Check sheet for the modelled part. Datum: model origin and axes. Units: mm. Round coordinates to 2 decimals unless told otherwise and drop trailing zeros. Order: outer loops, then holes, each group sorted by start corner. A loop starts at its lowest first (then second) coordinate and runs counter-clockwise, first axis right, second up. Notation, with made-up numbers: (-6, 22.5) -> (9, 22.5) arc R24 cw to (9, 32.5) -> close; hole circle Ø11 at (84, 21). An arc over 180 degrees is marked (long way). Answer in a Markdown table with one row per item. Add a question column.
1. Material ranges on L1, parallel to Y at x = -39.15, z = 0; L2, parallel to Z at x = -40.1, y = 9.75; L3, parallel to Y at x = -39.35, z = -31.5, recorded low to high. Write a range as from..to.
2. Sectioned sample at C-C, the plane z = 34. Count the separate pieces of the cut face and the enclosed holes in it, then the cut area to 3 significant figures.
3. Sectioned sample at A-A, the plane y = 9.75. Record the boundary of the cut face in (x, z), then the cut area to 3 significant figures.
4. Draft check along Y on faces 1 (the cylindrical face through (-39.532, 40.124, -47.641)), 2 (the cylindrical face through (-39.53, 4.97, 8.1)), 3 (the flat face through (-38.053, -2, -1)). Enter one of: +Y half, -Y half, draft (parallel to the pull), parting line (faces both ways), or undercut.
5. Depth check by flat-ended pin: P1, Ø4, axis at y = 3.39, z = -6.36, coming from the -X side; P2, Ø1.5, axis at x = -38.5, y = 29, coming from the -Z side; P3, Ø1.5, axis at x = -40.5, z = 26, coming from the +Y side. Enter the tip coordinate at first touch or a pass-through.
6. Sectioned sample at B-B, the plane z = 0. Record the boundary of the cut face in (x, y), then the cut area to 3 significant figures.
```python
from build123d import *

# Parameters (mm, degrees)
SKIZZE1_W                        = 3
SKIZZE1_H                        = 52.95
F_4_7_4_7_DURCHMESSER_BOHRUNG1_D = 4.7
SKIZZE5_RX                       = 25
SKIZZE5_RY                       = 10
SCHNITT_LINEAR_AUSTRAGEN1_DEPTH  = 3
KREISMUSTER1_COUNT               = 4


with BuildPart() as part:
    # Skizze1 → Rotation1 (revolve)
    with BuildSketch(Plane.XY):
        with Locations((-39.553372853, 39.775)):
            Rectangle(SKIZZE1_W, SKIZZE1_H)
    revolve(axis=Axis((-17.6629112, 9.75, 0), (-1, 0, 0)))

    # Ø4.7 (4.7) Durchmesser Bohrung1 (through all)
    with Locations(Plane(origin=(-41.053372853, 11.968723204, 19.868936148), x_dir=(0, 0, 1), z_dir=(-1, 0, 0))):
        with Locations((-13.504975118, -8.582684234), (-26.232897179, -8.582684234), (-26.232897179, 4.145237827), (-13.504975118, 4.145237827)):
            Hole(F_4_7_4_7_DURCHMESSER_BOHRUNG1_D / 2)

    # Skizze5 → Schnitt-Linear austragen1 (cut)
    with BuildSketch(Plane(origin=(-38.053372853, 0, 0), x_dir=(0, 0, -1), z_dir=(1, 0, 0))):
        with Locations(Location((-23.027329597, 32.684515508), (0, 0, 45.090609512))):
            Ellipse(SKIZZE5_RX, SKIZZE5_RY)
    schnitt_linear_austragen1 = extrude(amount=-SCHNITT_LINEAR_AUSTRAGEN1_DEPTH, mode=Mode.SUBTRACT)

    # Kreismuster1: Schnitt-Linear austragen1 ×4 about axis
    kreismuster1_axis = Axis((0, 9.75, 0), (-1, 0, 0))
    for i in range(1, KREISMUSTER1_COUNT):
        add(schnitt_linear_austragen1.rotate(kreismuster1_axis, i * 360 / KREISMUSTER1_COUNT), mode=Mode.SUBTRACT)


solid = part.part
```
Answer key:
| question | item | result |
|---|---|---|
| 1 | L1 | y = -46.75..6.2, 13.3..66.25 |
| 1 | L2 | z = -56.5..-3.55, 3.55..56.5 |
| 1 | L3 | y = -37.15..-18.8, 4.73..14.87, 38.31..56.65 |
| 2 | separate pieces | 3 |
| 2 | enclosed holes | 0 |
| 2 | area | 142 mm² |
| 3 | outline | (-41.05, -56.5) -> (-38.05, -56.5) -> (-38.05, -3.55) -> (-41.05, -3.55) -> close; (-41.05, 3.55) -> (-38.05, 3.55) -> (-38.05, 56.5) -> (-41.05, 56.5) -> close |
| 3 | area | 318 mm² |
| 4 | face 1 | parting line |
| 4 | face 2 | undercut |
| 4 | face 3 | draft |
| 5 | P1 | passes through |
| 5 | P2 | stops at z = -53.39 |
| 5 | P3 | stops at y = 60.29 |
| 6 | outline | (-41.05, -46.75) -> (-38.05, -46.75) -> (-38.05, 6.2) -> (-41.05, 6.2) -> close; (-41.05, 13.3) -> (-38.05, 13.3) -> (-38.05, 66.25) -> (-41.05, 66.25) -> close |
| 6 | area | 318 mm² |
